Check sheet for the modelled part. Datum: model origin and axes. Units: mm. A direction names the side the tool comes from. Round coordinates to 2 decimals unless told otherwise and drop trailing zeros. Write each loop counter-clockwise with the first axis right and the second up, starting at its lowest first coordinate (ties: lowest second). Pieces come first, ordered by that corner, then holes. Notation, with made-up numbers: M -31,21.25 L 3,21.25 A7 cw 3,34.25 Z; hole C 75.25,51.5 d1. An arc over 180 degrees is marked long. Put each result on its own line as item: value.
```python
from build123d import *

# Parameters (mm, degrees)
SKETCH1_R           = 24.5
BOSS_EXTRUDE1_DEPTH = 36
CUT_EXTRUDE1_DEPTH  = 12
CUT_EXTRUDE2_START  = -10
SKETCH3_R           = 24.5
SKETCH3_R_2         = 24
CUT_EXTRUDE2_DEPTH  = 3
CUT_EXTRUDE3_START  = -23
SKETCH4_R           = 24.5
SKETCH4_R_2         = 24
CUT_EXTRUDE3_DEPTH  = 3


with BuildPart() as part:
    # Sketch1 → Boss-Extrude1 (new body)
    with BuildSketch(Plane.XY):
        Circle(SKETCH1_R)
    extrude(amount=BOSS_EXTRUDE1_DEPTH)

    # Sketch2 → Cut-Extrude1 (cut)
    with BuildSketch(Plane.XY.offset(36)):
        Polygon((8.343860018, 8.343860018), (-3.054064732, 11.39792475), (-11.39792475, 3.054064732), (-8.343860018, -8.343860018), (3.054064732, -11.39792475), (11.39792475, -3.054064732), align=None)
    extrude(amount=-CUT_EXTRUDE1_DEPTH, mode=Mode.SUBTRACT)

    # Sketch3 → Cut-Extrude2 (cut)
    with BuildSketch(Plane.XY.offset(36).offset(CUT_EXTRUDE2_START)):
        Circle(SKETCH3_R)
        Circle(SKETCH3_R_2, mode=Mode.SUBTRACT)
    extrude(amount=-CUT_EXTRUDE2_DEPTH, mode=Mode.SUBTRACT)

    # Sketch4 → Cut-Extrude3 (cut)
    with BuildSketch(Plane.XY.offset(36).offset(CUT_EXTRUDE3_START)):
        Circle(SKETCH4_R)
        Circle(SKETCH4_R_2, mode=Mode.SUBTRACT)
    extrude(amount=-CUT_EXTRUDE3_DEPTH, mode=Mode.SUBTRACT)


solid = part.part
```
1. Access from +Z, -Z, +X, -X, +Y, -Y to the whole of each face (thin tool, end or side, straight path). Record for faces 1 (the flat face through (16.2, -18, 23)), 2 (the cylindrical face through (13.17, 20.66, 4.93)), 3 (the flat face through (0, 0, 24)).
Computed values:
face 1: none
face 2: +Z, -Z
face 3: +Z
2. Release check for a two-part mould opening along Z. For faces 4 (the flat face through (11, 0, 36)), 5 (the flat face through (-2.72, -9.85, 30.08)), 6 (the flat face through (16.2, -18, 13)), 7 (the cylindrical face through (-23.977, 1.055, 24.521)) record: +Z half, -Z half, draft (parallel to the pull), parting line (faces both ways), or undercut.
Computed values:
face 4: +Z half
face 5: draft
face 6: undercut
face 7: undercut
3. Cross-section at B-B (x = 0). Enter the section's corners in (y, z), then the cut area to 3 significant figures.
Computed values:
outline: M -24.5,0 L 24.5,0 L 24.5,10 L 24,10 L 24,13 L 24.5,13 L 24.5,23 L 24,23 L 24,26 L 24.5,26 L 24.5,36 L 10.58,36 L 10.58,24 L -10.58,24 L -10.58,36 L -24.5,36 L -24.5,26 L -24,26 L -24,23 L -24.5,23 L -24.5,13 L -24,13 L -24,10 L -24.5,10 Z
area: 1,500 mm2
4. Scan lines: probe 1 along Z at (x, y) = (23.5, -5.5); probe 2 along X at (y, z) = (2.5, 30.5); probe 3 along Y at (x, z) = (-5, 28). Record each from-to range of solid material in increasing order.
Computed values:
probe 1: z = 0 to 10, 13 to 23, 26 to 36
probe 2: x = -24.37 to -11.25, 9.91 to 24.37
probe 3: y = -23.98 to -9.24, 9.45 to 23.98
5. Cross-section at D-D (x = 20.5). Enter the section's corners in (y, z), then the cut area to 3 significant figures.
Computed values:
outline: M -13.42,0 L 13.42,0 L 13.42,10 L 12.48,10 L 12.48,13 L 13.42,13 L 13.42,23 L 12.48,23 L 12.48,26 L 13.42,26 L 13.42,36 L -13.42,36 L -13.42,26 L -12.48,26 L -12.48,23 L -13.42,23 L -13.42,13 L -12.48,13 L -12.48,10 L -13.42,10 Z
area: 955 mm2
6. Cross-section at C-C (y = 4). Enter the section's corners in (x, z).
Computed values:
outline: M -24.17,0 L 24.17,0 L 24.17,10 L 23.66,10 L 23.66,13 L 24.17,13 L 24.17,23 L 23.66,23 L 23.66,26 L 24.17,26 L 24.17,36 L 9.51,36 L 9.51,24 L -10.45,24 L -10.45,36 L -24.17,36 L -24.17,26 L -23.66,26 L -23.66,23 L -24.17,23 L -24.17,13 L -23.66,13 L -23.66,10 L -24.17,10 Z
7. Depth check by flat-ended pin: pin 1 Ø5 at (x, y) = (-1.5, -15.5) entering from -Z; pin 2 Ø3 at (y, z) = (-19, 16) entering from -X; pin 3 Ø1 at (x, z) = (-15, 26.5) entering from +Y; pin 4 Ø7 at (x, y) = (5.5, -3) entering from +Z. Enter the tip coordinate at first touch or a pass-through.
Computed values:
pin 1: stops at z = 0
pin 2: stops at x = -17.15
pin 3: stops at y = 19.75
pin 4: stops at z = 24
8. Cross-section at A-A (z = 27). Enter the section's corners in (x, y).
Computed values:
outline: C 0,0 d49; hole M -11.4,3.05 L -8.34,-8.34 L 3.05,-11.4 L 11.4,-3.05 L 8.34,8.34 L -3.05,11.4 Z
